```python
from build123d import *

# Parameters (mm, degrees)
CYLINDER003_R       = 2
CYLINDER003_DEPTH   = 10
BOX_W               = 2
BOX_H               = 10
BOX_DEPTH           = 10
SKETCH003_R         = 2.25
PAD003_DEPTH        = 2
PAD002_DEPTH        = 18
CUT_PLACEMENT_ANGLE = 180


with BuildPart() as cylinder003:
    # Cylinder003 → Cylinder003 (new body)
    with BuildSketch(Plane(origin=(0, 43, -22), x_dir=(1, 0, 0), z_dir=(0, 0, 1))):
        Circle(CYLINDER003_R)
    extrude(amount=CYLINDER003_DEPTH)


with BuildPart() as cube:
    # Box → Box (new body)
    with BuildSketch(Plane(origin=(-1, -58, -13), x_dir=(1, 0, 0), z_dir=(0, 0, 1))):
        with Locations((1, 5)):
            Rectangle(BOX_W, BOX_H)
    extrude(amount=BOX_DEPTH)


with BuildPart() as body003:
    # Sketch003 → Pad003 (new body)
    with BuildSketch(Plane.XY):
        with BuildLine():
            ThreePointArc((30.15435, 22.5), (0, 52.65435), (-30.15435, 22.5))
            Line((-30.15435, 22.5), (-30.15435, -22.5))
            ThreePointArc((-30.15435, -22.5), (0, -52.65435), (30.15435, -22.5))
            Line((30.15435, 22.5), (30.15435, -22.5))
        make_face()
        with Locations((0, 27)):
            Circle(SKETCH003_R, mode=Mode.SUBTRACT)
        with Locations((0, -23)):
            Circle(SKETCH003_R, mode=Mode.SUBTRACT)
    extrude(amount=PAD003_DEPTH)


with BuildPart() as body003_1:
    # Body003 placement: moved
    add(body003.part.moved(Location((0, 0, -18))))


with BuildPart() as f_65_trafficlightcasebottom:
    # Sketch002 → Pad002 (new body)
    with BuildSketch(Plane.XY):
        with BuildLine():
            ThreePointArc((32.15435, 22.5), (0, 54.65435), (-32.15435, 22.5))
            Line((-32.15435, 22.5), (-32.15435, -22.5))
            ThreePointArc((-32.15435, -22.5), (0, -54.65435), (32.15435, -22.5))
            Line((32.15435, 22.5), (32.15435, -22.5))
        make_face()
        with BuildLine():
            ThreePointArc((30.15435, 22.5), (0, 52.65435), (-30.15435, 22.5))
            Line((-30.15435, 22.5), (-30.15435, -22.5))
            ThreePointArc((-30.15435, -22.5), (0, -52.65435), (30.15435, -22.5))
            Line((30.15435, 22.5), (30.15435, -22.5))
        make_face(mode=Mode.SUBTRACT)
    extrude(amount=PAD002_DEPTH)


with BuildPart() as f_65_trafficlightcasebottom_1:
    # Body002 placement: moved
    add(f_65_trafficlightcasebottom.part.moved(Location((0, 0, -18))))

    # Fusion001: union Body003
    add(body003_1.part)

    # Cut: cut Cube
    add(cube.part, mode=Mode.SUBTRACT)


with BuildPart() as f_65_trafficlightcasebottom_2:
    # Cut placement: moved
    add(f_65_trafficlightcasebottom_1.part.rotate(Axis((0, 0, 0), (0, 0, 1)), CUT_PLACEMENT_ANGLE))

    # Cut005: cut Cylinder003
    add(cylinder003.part, mode=Mode.SUBTRACT)


solid = f_65_trafficlightcasebottom_2.part
```
Here's how the part is built. I have some questions about the finished solid (model axes, mm). A direction names the side the tool comes from. Give positions to 0.01 mm unless a question says otherwise; leave off trailing zeros. Order: outer loops, then holes, each group sorted by start corner. A loop starts at its lowest first (then second) coordinate and runs counter-clockwise, first axis right, second up. Notation, with made-up numbers: (77, 31.5) - (91, 31.5) arc R14 ccw to (91, 42.5) - close; hole circle Ø3 at (32, -32). An arc over 180 degrees is marked (long way). Answer as a JSON object with one key per item and string values. Group by question number.
Item 1: If we section it at D-D on x = -5: Please give me the cut outline in (y, z), and give its area (3 significant figures).
Item 2: If we mould it in two halves opening along X, with no side actions, what happens to faces 1 (the cylindrical face through (0.707, 54.647, -15.126)), 2 (the cylindrical face through (0.488, 25.196, -17.014)), 3 (the flat face through (0, -1, -16)), 4 (the flat face through (0, -1, -18))? For each: pulls with the +X half, pulls with the -X half, needs draft (parallel to the pull), parting line crosses it, or undercut.
Item 3: Please list where these lines run through material, in increasing order: probe 1 along Y at (x, z) = (0, -17.15); probe 2 along X at (y, z) = (21, -12.75); probe 3 along X at (y, z) = (23, -16.9).
Item 4: If we section it at B-B on y = 43: Please give me the cut outline in (x, z).
Item 5: For P1, Ø3, axis at y = 25.5, z = -9.5, coming from the +X side; P2, Ø1, axis at x = 6.5, y = 24, coming from the +Z side; P3, Ø2.5, axis at x = 0, y = 43, coming from the -Z side (1 decimal); P4, Ø5, axis at x = -1.5, z = -6, coming from the -Y side, each with a flat end and sliding along its axis, tell me the tip position at first contact or that it passes through.
Item 6: If we section it at C-C on z = -8.5: Please give me the cut outline in (x, y), and give its area (3 significant figures).
Item 7: If we section it at A-A on y = 5.5: Please give me the cut outline in (x, z).
Item 8: Which directions (+Z, -Z, +X, -X, +Y, -Y) give clear straight access to the entire face, cutting with the end or side of a thin tool? Please do faces 5 (the flat face through (-32.154, 0, -9)), 6 (the flat face through (-1, 54, -8)), 7 (the cylindrical face through (0.663, 52.647, -2.779)).
Result set:
{
 "1": {"outline": "(-54.26, -18) - (54.26, -18) - (54.26, 0) - (52.24, 0) - (52.24, -16) - (-52.24, -16) - (-52.24, 0) - (-54.26, 0) - close", "area": "282 mm²"},
 "2": {"face 1": "parting line crosses it", "face 2": "undercut", "face 3": "undercut", "face 4": "needs draft"},
 "3": {"probe 1": "-54.65 to -29.25, -24.75 to 20.75, 25.25 to 41, 45 to 54.65", "probe 2": "-32.15 to -30.15, 30.15 to 32.15", "probe 3": "-32.15 to -2.25, 2.25 to 32.15"},
 "4": {"outline": "(-24.77, -18) - (-2, -18) - (-2, -16) - (-22.11, -16) - (-22.11, 0) - (-24.77, 0) - close; (2, -18) - (24.77, -18) - (24.77, 0) - (22.11, 0) - (22.11, -16) - (2, -16) - close"},
 "5": {"P1": "x = 32.12", "P2": "z = -16", "P3": "through", "P4": "y = -54.65"},
 "6": {"outline": "(-32.15, -22.5) arc R32.15 ccw to (32.15, -22.5) - (32.15, 22.5) arc R32.15 ccw to (1, 54.64) - (1, 52.64) arc R30.15 cw to (30.15, 22.5) - (30.15, -22.5) arc R30.15 cw to (-30.15, -22.5) - (-30.15, 22.5) arc R30.15 cw to (-1, 52.64) - (-1, 54.64) arc R32.15 ccw to (-32.15, 22.5) - close", "area": "567 mm²"},
 "7": {"outline": "(-32.15, -18) - (32.15, -18) - (32.15, 0) - (30.15, 0) - (30.15, -16) - (-30.15, -16) - (-30.15, 0) - (-32.15, 0) - close"},
 "8": {"face 5": "+Z, -Z, -X, +Y, -Y", "face 6": "+Y", "face 7": "+Z"}
}
